from build123d import *

# Parameters (mm, degrees)
F0_R      = 44.45
F1_DEPTH  = 6.35
F2_R      = 16.7386
F3_DEPTH  = 6.35
F7_R      = 2.159
F8_DEPTH  = 6.35
F9_R      = 2.159
F10_DEPTH = 6.35


with BuildPart() as f1:
    # F0 (on Top) → F1 (new body)
    with BuildSketch(Plane.XY):
        Circle(F0_R)
    extrude(amount=F1_DEPTH)

    # F2 (on face) → F3 (cut)
    with BuildSketch(Plane.XY.offset(6.35)):
        Circle(F2_R)
    extrude(amount=-F3_DEPTH, mode=Mode.SUBTRACT)

    # F7 (on face) → F8 (cut)
    with BuildSketch(Plane.XY.offset(6.35)):
        with Locations((-18.529808, 15.005284)):
            Circle(F7_R)
    extrude(amount=-F8_DEPTH, mode=Mode.SUBTRACT)

    # F9 (on face) → F10 (cut)
    with BuildSketch(Plane.XY.offset(6.35)):
        with Locations((18.525945, -14.854639)):
            Circle(F9_R)
    extrude(amount=-F10_DEPTH, mode=Mode.SUBTRACT)


solid = f1.part
Read the model definition and answer for the solid it produces. Units are mm, in the model's axes. Coordinates: 2 decimals unless noted, no trailing zeros. Loops run counter-clockwise (first coordinate to the right, second up) from the corner with the lowest first, then second, coordinate; pieces in that order, holes last. Notation, with made-up numbers: (54, -2) - (68, -2) arc R27 cw to (68, 26) - close; hole circle Ø8 at (0.25, -23.5). An arc over 180 degrees is marked (long way). Answer in a Markdown table with one row per item.
Q1. Find section D-D on y = -30. Write down the section's boundary in (x, z), plus the area to 3 significant figures.
Here are the results:
| item | result |
|---|---|
| outline | (-32.8, 0) - (32.8, 0) - (32.8, 6.35) - (-32.8, 6.35) - close |
| area | 417 mm^2 |
Q2. Straight lines are drawn through the part: line 1 along Y through (x, z) = (0, 2.75); line 2 along Y through (x, z) = (9.5, 1); line 3 along X through (y, z) = (6, 4.25). For each, find the intervals that lie inside material, in ascending order. Write a range as [from, to].
Here are the results:
| item | result |
|---|---|
| line 1 | y = [-44.45, -16.74], [16.74, 44.45] |
| line 2 | y = [-43.42, -13.78], [13.78, 43.42] |
| line 3 | x = [-44.04, -15.63], [15.63, 44.04] |
Q3. Find section C-C on z = 2.25. Write down the section's boundary in (x, y).
Here are the results:
| item | result |
|---|---|
| outline | circle Ø88.9 at (0, 0); hole circle Ø4.32 at (-18.53, 15.01); hole circle Ø33.48 at (0, 0); hole circle Ø4.32 at (18.53, -14.85) |
Q4. Given P1, Ø1, axis at y = 25, z = 1, coming from the +X side; P2, Ø1, axis at x = 7, z = 4.5, coming from the +Y side, each flat-ended and moving along its own axis, determine where each tip first touches the part or whether it passes through.
Here are the results:
| item | result |
|---|---|
| P1 | stops at x = 37.09 |
| P2 | stops at y = 43.97 |
Q5. Find section A-A on x = 0. Write down the section's boundary in (y, z), plus the area to 3 significant figures.
Here are the results:
| item | result |
|---|---|
| outline | (-44.45, 0) - (-16.74, 0) - (-16.74, 6.35) - (-44.45, 6.35) - close; (16.74, 0) - (44.45, 0) - (44.45, 6.35) - (16.74, 6.35) - close |
| area | 352 mm^2 |
Q6. The mould has two halves that part along X. Classify faces 1 (the cylindrical face through (-13.28, -10.19, 3.22)), 2 (the cylindrical face through (42.397, 13.352, 3.131)), 3 (the flat face through (-1, -19, 0)): pulls with the +X half, pulls with the -X half, needs draft (parallel to the pull), parting line crosses it, or undercut.
Here are the results:
| item | result |
|---|---|
| face 1 | undercut |
| face 2 | parting line crosses it |
| face 3 | needs draft |
